Autodesk Inventor part; units mm, degrees
ref_plane "Work Plane1" through (29, 0, 0) normal (0, -1, 0) x (1, 0, 0)
ref_plane "YZ Plane" through (0, 0, 0) normal (1, 0, 0) x (0, 1, 0)
ref_plane "XZ Plane" through (0, 0, 0) normal (0, 1, 0) x (-1, 0, 0)
sketch "Sketch1" plane through (0, 0, 0) normal (0, 0, 1) x (1, 0, 0)
  line L0 (-1.7103, 0) -> (15.875, 0)
  line L1 (15.875, 0) -> (15.875, 3.175)
  line L2 (15.875, 3.175) -> (3.1752, 3.175)
  line L3 (3.1752, 3.175) -> (0.0001, 3.175)
  line L4 (0.0001, 3.175) -> (0, 3.175)
  line L5 (0, 3.175) -> (0, 4.7625)
  line L6 (0, 4.7625) -> (-6.35, 4.7625)
  line L7 (-6.35, 4.7625) -> (-6.35, 2.757)
  line L8 (-6.35, 2.757) -> (-3.302, 2.757)
  line L9 (-3.302, 2.757) -> (-1.7103, 0)
  line L10 (-10.795, 0) -> (20.32, 0)
  line L11 (0, -0.9525) -> (0, 5.715)
  line L12 (3.1752, 3.175) -> (0, 3.175) construction
  dimension "d1" = 12.6998
  dimension "d2" = 3.1751
  dimension "d3" = 6.35
  dimension "d4" = 3.048
  dimension "d5" = 60
  dimension "d6" = 6.35
  dimension "d7" = 6.35
  dimension "d8" = 5.5139
  dimension "d9" = 9.525
  dimension "d26" = 15.875
revolve "Body" add sketch "Sketch1" angle 360 about axis through (-1.7103, 0, 0) along (1, 0, 0)
sketch "Sketch2" plane through (-6.35, 0, 0) normal (-1, 0, 0) x (0, 0, 1)
  circle A0 centre (0, 0) radius 2.757
  line L0 (0, -6.6675) -> (0, 6.6675)
  line L1 (-6.6675, 0) -> (6.6675, 0)
  line L2 (2.757, 0) -> (1.3785, -2.3876)
  line L3 (1.3785, -2.3876) -> (-1.3785, -2.3876)
  line L4 (-1.3785, -2.3876) -> (-2.757, 0)
  line L5 (-2.757, 0) -> (-1.3785, 2.3876)
  line L6 (-1.3785, 2.3876) -> (1.3785, 2.3876)
  line L7 (1.3785, 2.3876) -> (2.757, 0)
extrude "Slot" add sketch "Sketch2" against normal up to next contours L7 A0 | A0 L2 | L6 L0 A0 | A0 L0 L3 | L0 L6 A0 | A0 L3 L0 | L4 A0 | A0 L5
fillet "Fillet1" radius 0.635 1 edges at (-6.35, -4.7625, 0)
thread "Thread"
chamfer "Chamfer1" distance 0.7556 distance2 0.7556 1 edges at (15.875, -3.175, 0) measured on face at (15.875, 0.0983, -0.8099)
ref_plane "Work Plane1" through (29, 0, 0) normal (0, -1, 0) x (1, 0, 0)
fillet "Fillet2" radius 0.1778 1 edges at (0.0001, -3.175, 0)
equation "\"d30\" = R"
equation "\"d17\" = RR"
equation "\"d13\" = GEL"
equation "\"d15\" = -0.5 * SPD + 0.5 * GD"
equation "\"d16\" = GUL"
equation "\"d1\" = GEL"
equation "\"d3\" = KOH"
equation "\"d4\" = INTI"
equation "\"d6\" = GD"
equation "\"d7\" = BDM"
equation "\"d8\" = 1.1547 * SW"
equation "\"d9\" = KOD"
equation "\"d26\" = NLG"
equation "\"GD\" = 6.35"
equation "\"NLG\" = 15.875"
equation "\"GEL\" = 12.6998"
equation "\"KOD\" = 9.525"
equation "\"KOH\" = 6.35"
equation "\"INTI\" = 3.048"
equation "\"GAL\" = 3.175"
equation "\"GUL\" = 0.75565"
equation "\"BDM\" = 6.35"
equation "\"SW\" = 4.7752"
equation "\"RR\" = 0.635"
equation "\"SPD\" = 4.8387"
equation "\"R\" = 0.1778"
equation "\"PHH\" = 0.2032"
equation "\"GD1\" = SPD"
equation "\"THREADDIA\" = 6.35"
equation "\"FAWI\" = 45deg"
equation "\"KOH1\" = 5.715"
equation "\"NND\" = 6.35"
equation "\"TOA\" = 30deg"
equation "\"E0\" = 1.155 * SW"
properties part number "ANSI B18.3 - 1/4 - 20 UNC - 5/8 HS HCS" material "Steel, Mild"
Design review of the part built by this model. Coordinates are the model's own, in mm. A direction names the side the tool comes from. Round coordinates to 2 decimals unless told otherwise and drop trailing zeros. One line per question, with ' | ' between items.
(1) Machinability: for faces 1 (the conical face through (0, -3, 2)), 2 (the flat face through (-6.35, -2, 2)), 3 (the flat face through (-4.74, 1.21, 2.06)), which of the approach directions +Z, -Z, +X, -X, +Y, -Y give a long, thin tool a straight path to every point of the face, cutting with its end or side? Answer none if there is none.
Result sheet:
face 1: +X | face 2: +Z, -Z, -X, +Y, -Y | face 3: -X
(2) Wall thickness on line 1 (X direction, y = -1.5, z = 1) (3 decimals); line 2 (X direction, y = -0.25, z = -3.5); line 3 (Z direction, x = -5, y = 0.5): over which ranges is each line inside the solid? List them lowest first. Write a range as [from, to].
Result sheet:
line 1: [-2.751, 15.875] | line 2: [-6.35, 0] | line 3: [-4.74, -2.47], [2.47, 4.74]
(3) Insertion check: P1, Ø1.5, axis at x = 12.5, z = -2, coming from the -Y side; P2, Ø1.5, axis at x = 9.5, y = 2.5, coming from the +Z side; P3, Ø4, axis at x = 10, z = -1, coming from the -Y side (3 decimals). Each pin has a flat end and moves straight along its axis. Give the tip position at first contact, or say it passes through.
Result sheet:
P1: y = -2.92 | P2: z = 2.65 | P3: y = -3.175
(4) Draft analysis for pull direction Y (two halves, no side actions). For faces 4 (the cylindrical face through (-2.9, -3.78, 2.9)), 5 (the flat face through (-5, 2.388, 0)), 6 (the flat face through (15.875, 0, 0)), 7 (the conical face through (-1.81, 0.165, -0.052)), state which applies: released by +Y, released by -Y, zero draft, split by the parting line, or undercut.
Result sheet:
face 4: split by the parting line | face 5: undercut | face 6: zero draft | face 7: undercut
